from build123d import *

# Parameters (mm, degrees)
SKETCH1_R           = 22.5
SKETCH1_R_2         = 2.15
BOSS_EXTRUDE1_DEPTH = 5
SKETCH2_R           = 3.75
CUT_EXTRUDE1_DEPTH  = 4
BOSS_EXTRUDE2_DEPTH = 1
BOSS_EXTRUDE3_DEPTH = 7
FILLET1_R           = 1


# Read off the part's stored shape, not the designer's step: Boss-Extrude2
with BuildPart() as part:
    # Sketch1 → Boss-Extrude1 (new body)
    with BuildSketch(Plane.XY.offset(31)):
        Circle(SKETCH1_R)
        with Locations((-6, 10.392304845)):
            Circle(SKETCH1_R_2, mode=Mode.SUBTRACT)
        with Locations((-6, -10.392304845)):
            Circle(SKETCH1_R_2, mode=Mode.SUBTRACT)
        with Locations((12, 0)):
            Circle(SKETCH1_R_2, mode=Mode.SUBTRACT)
    extrude(amount=BOSS_EXTRUDE1_DEPTH)

    # Sketch2 → Cut-Extrude1 (cut)
    with BuildSketch(Plane.XY.offset(36)):
        with Locations((-6, 10.392304845)):
            Circle(SKETCH2_R)
        with Locations((12, 0)):
            Circle(SKETCH2_R)
        with Locations((-6, -10.392304845)):
            Circle(SKETCH2_R)
    extrude(amount=-CUT_EXTRUDE1_DEPTH, mode=Mode.SUBTRACT)

    # Boss-Extrude2 outline → Boss-Extrude2 (add)
    with BuildSketch(Plane.XY.offset(36)):
        with BuildLine():
            ThreePointArc((9.174479167, -2.46554903), (8.25, 0), (9.174479167, 2.46554903))
            ThreePointArc((9.174479167, 2.46554903), (4.75, 8.227241336), (-2.452011489, 9.17810654))
            ThreePointArc((-2.452011489, 9.17810654), (-4.125, 7.144709581), (-6.722467678, 6.712557509))
            ThreePointArc((-6.722467678, 6.712557509), (-9.5, 0), (-6.722467678, -6.71255751))
            ThreePointArc((-6.722467678, -6.71255751), (-4.125, -7.144709581), (-2.452011489, -9.17810654))
            ThreePointArc((-2.452011489, -9.17810654), (4.75, -8.227241336), (9.174479167, -2.46554903))
        make_face()
    extrude(amount=BOSS_EXTRUDE2_DEPTH)

    # Sketch4 → Boss-Extrude3 (add)
    with BuildSketch(Plane.XY.offset(37)):
        with BuildLine():
            ThreePointArc((8.424479167, -1.130553303), (8.25, 0), (8.424479167, 1.130553303))
            ThreePointArc((8.424479167, 1.130553303), (4.25, 7.361215932), (-3.233151703, 7.861089623))
            ThreePointArc((-3.233151703, 7.861089623), (-4.125, 7.144709581), (-5.191327464, 6.730536321))
            ThreePointArc((-5.191327464, 6.730536321), (-8.5, 0), (-5.191327464, -6.730536321))
            ThreePointArc((-5.191327464, -6.730536321), (-4.125, -7.144709581), (-3.233151703, -7.861089623))
            ThreePointArc((-3.233151703, -7.861089623), (4.25, -7.361215932), (8.424479167, -1.130553303))
        make_face()
    extrude(amount=BOSS_EXTRUDE3_DEPTH)

    # Fillet1
    # the kernel refuses this fillet: 1 mm, written as the material it takes off along each edge
    with BuildSketch(Plane(origin=(9.174479167, -2.46554903, 36), x_dir=(-0.2868427193714439, -0.9579776898986714, 0), z_dir=(0, 0, 1)), Plane(origin=(-2.452011489, 9.17810654, 36), x_dir=(0.9730543753959973, 0.23057576308603095, 0), z_dir=(0, 0, 1)), Plane(origin=(-6.722467678, -6.71255751, 36), x_dir=(-0.6862116560068084, 0.7274019268330224, 0), z_dir=(0, 0, 1))) as fillet1_piece_1:
        with BuildLine():
            CenterArc((0.510994589, -0.999596963), FILLET1_R, 88.373235151, 52.473151254)
            ThreePointArc((-0.264461334, -0.368195259), (-0.126661785, -0.188097556), (0, 0))
            ThreePointArc((0, 0), (0.269691589, 0.003828853), (0.539383177, 0))
        make_face()
    extrude(amount=2.348457943, mode=Mode.SUBTRACT)
    with BuildSketch(Plane(origin=(9.174479167, 2.46554903, 36), x_dir=(-0.28684271937144556, 0.957977689898671, 0), z_dir=(0, 0, 1)), Plane(origin=(-2.452011489, -9.17810654, 36), x_dir=(0.9730543753972882, -0.23057576308058297, 0), z_dir=(0, 0, 1))) as fillet1_piece_2:
        with BuildLine():
            CenterArc((0.510994589, 0.999596963), FILLET1_R, 219.153613594, 52.473151254)
            ThreePointArc((-0.264461334, 0.368195259), (-0.126661785, 0.188097556), (0, 0))
            ThreePointArc((0, 0), (0.269691589, -0.003828853), (0.539383177, 0))
        make_face()
    extrude(amount=2.348457943, mode=Mode.SUBTRACT)
    with BuildSketch(Plane(origin=(-6.722467678, 6.712557509, 36), x_dir=(-0.686211656019457, -0.72740192682109, 0), z_dir=(0, 0, 1))) as fillet1_piece_3:
        with BuildLine():
            CenterArc((0.510994589, 0.999596963), FILLET1_R, 219.153613615, 52.473151233)
            ThreePointArc((-0.264461334, 0.368195259), (-0.126661785, 0.188097556), (0, 0))
            ThreePointArc((0, 0), (0.269691588, -0.003828853), (0.539383177, 0))
        make_face()
    extrude(amount=2.348457942, mode=Mode.SUBTRACT)
    with BuildSketch(Plane(origin=(8.424479167, -1.130553303, 37), x_dir=(-0.27697269239961747, 0.9608777901819289, 0), z_dir=(0, 0, 1)), Plane(origin=(-3.233151703, 7.861089623, 37), x_dir=(-0.6936582300297728, -0.7203042828638206, 0), z_dir=(0, 0, 1)), Plane(origin=(-5.191327464, -6.730536321, 37), x_dir=(0.9706309224297027, -0.24057350731795996, 0), z_dir=(0, 0, 1))) as fillet1_piece_4:
        with BuildLine():
            CenterArc((0.217604369, 0.999672253), FILLET1_R, 244.726311149, 23.806727181)
            ThreePointArc((-0.20933828, 0.095393549), (-0.104991878, 0.046988536), (0, 0))
            ThreePointArc((0, 0), (0.096001927, 0.001229051), (0.192003855, 0))
        make_face()
    extrude(amount=7.57512197, mode=Mode.SUBTRACT)
    with BuildSketch(Plane(origin=(8.424479167, 1.130553303, 37), x_dir=(-0.27697269239961625, -0.9608777901819292, 0), z_dir=(0, 0, 1)), Plane(origin=(-5.191327464, 6.730536321, 37), x_dir=(0.9706309224296972, 0.24057350731798183, 0), z_dir=(0, 0, 1)), Plane(origin=(-3.233151703, -7.861089623, 37), x_dir=(-0.6936582300297843, 0.7203042828638094, 0), z_dir=(0, 0, 1))) as fillet1_piece_5:
        with BuildLine():
            CenterArc((0.217604369, -0.999672253), FILLET1_R, 91.46696167, 23.806727181)
            ThreePointArc((-0.20933828, -0.095393549), (-0.104991878, -0.046988536), (0, 0))
            ThreePointArc((0, 0), (0.096001927, -0.001229051), (0.192003855, 0))
        make_face()
    extrude(amount=7.57512197, mode=Mode.SUBTRACT)


solid = part.part
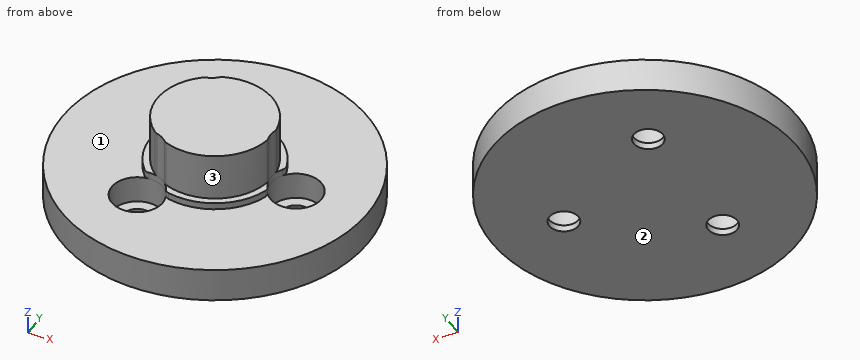
For this review, take the finished solid that the model builds, in its own axes (mm). Face numbers are marked on the shaded views. A direction names the side the tool comes from. Coordinates: 2 decimals unless noted, no trailing zeros. Order: outer loops, then holes, each group sorted by start corner. A loop starts at its lowest first (then second) coordinate and runs counter-clockwise, first axis right, second up. Notation, with made-up numbers: (-30.75, 68) -> (0.25, 68) arc R18 cw to (0.25, 83) -> close; hole circle Ø2 at (-24, 40.25). An arc over 180 degrees is marked (long way). Return JSON: item names as keys, results as strings.
1. We need section D-D on x = 12. Write out the cut boundary in (y, z), and give its area (3 significant figures).
Answer block:
{"outline": "(-19.03, 31) -> (-2.15, 31) -> (-2.15, 32) -> (-3.75, 32) -> (-3.75, 36) -> (-19.03, 36) -> close; (2.15, 31) -> (19.03, 31) -> (19.03, 36) -> (3.75, 36) -> (3.75, 32) -> (2.15, 32) -> close", "area": "156 mm²"}
2. We need section C-C on z = 40.5. Write out the cut boundary in (x, y), and give its area (3 significant figures).
Answer block:
{"outline": "(-5.37, -6.59) arc R1 ccw to (-5, -6.78) arc R3.75 cw to (-3.37, -7.72) arc R1 ccw to (-3.02, -7.95) arc R8.5 ccw to (8.39, -1.36) arc R1 ccw to (8.37, -0.95) arc R3.75 cw to (8.37, 0.95) arc R1 ccw to (8.39, 1.36) arc R8.5 ccw to (-3.02, 7.95) arc R1 ccw to (-3.37, 7.72) arc R3.75 cw to (-5, 6.78) arc R1 ccw to (-5.37, 6.59) arc R8.5 ccw to start", "area": "226 mm²"}
3. For line 1 (Y direction, x = -6, z = 35); line 2 (Y direction, x = -6, z = 31.7); line 3 (Z direction, x = 10, y = 13.5), list the stretches that pass through material, from the lowest coordinate up. Write a range as from..to.
Answer block:
{"line 1": "-21.69..-14.14, -6.64..6.64, 14.14..21.69", "line 2": "-21.69..-12.54, -8.24..8.24, 12.54..21.69", "line 3": "31..36"}
4. We need section B-B on x = 0. Write out the cut boundary in (y, z).
Answer block:
{"outline": "(-22.5, 31) -> (22.5, 31) -> (22.5, 36) -> (9.5, 36) -> (9.5, 37) -> (8.5, 37) -> (8.5, 44) -> (-8.5, 44) -> (-8.5, 37) -> (-9.5, 37) -> (-9.5, 36) -> (-22.5, 36) -> close"}
5. Machinability: for the marked faces 1, 2 and 3, which of the approach directions +Z, -Z, +X, -X, +Y, -Y give a long, thin tool a straight path to every point of the face, cutting with its end or side? Answer none if there is none.
Answer block:
{"face 1": "+Z", "face 2": "-Z, +X, -X, +Y, -Y", "face 3": "+Z, -Y"}
6. For pin 1 Ø4.5 at (x, y) = (12, 0) entering from +Z; pin 2 Ø4 at (x, z) = (-4, 39.5) entering from +Y; pin 3 Ø1 at (x, z) = (-11, 36) entering from -Y, all flat-tipped, find the tip position at first contact; note any pin that passes through.
Answer block:
{"pin 1": "z = 32", "pin 2": "y = 8.26", "pin 3": "y = -19.9"}
7. We need section A-A on y = 0. Write out the cut boundary in (x, z), and give its area (3 significant figures).
Answer block:
{"outline": "(-22.5, 31) -> (9.85, 31) -> (9.85, 32) -> (8.25, 32) -> (8.25, 44) -> (-8.5, 44) -> (-8.5, 37) -> (-9.5, 37) -> (-9.5, 36) -> (-22.5, 36) -> close; (14.15, 31) -> (22.5, 31) -> (22.5, 36) -> (15.75, 36) -> (15.75, 32) -> (14.15, 32) -> close", "area": "326 mm²"}
